from build123d import *

# Parameters (mm, degrees)
SKETCH1_W           = 95
SKETCH1_H           = 75
BOSS_EXTRUDE1_DEPTH = 32.5
SKETCH2_W           = 90
SKETCH2_H           = 70
CUT_EXTRUDE1_DEPTH  = 30
SKETCH3_R           = 1.75
BOSS_EXTRUDE2_DEPTH = 7
SKETCH4_R           = 1
BOSS_EXTRUDE3_DEPTH = 23
SKETCH5_W           = 52.348164398
SKETCH5_H           = 12
CUT_EXTRUDE2_DEPTH  = 7
FILLET1_R           = 2.5
FILLET2_R           = 2.5
FILLET3_R           = 2.5
FILLET4_R           = 2.5
FILLET5_R           = 2.5


with BuildPart() as part:
    # Sketch1 → Boss-Extrude1 (new body)
    with BuildSketch(Plane(origin=(0, 0, 0), x_dir=(1, 0, 0), z_dir=(0, 1, 0))):
        Rectangle(SKETCH1_W, SKETCH1_H)
    extrude(amount=BOSS_EXTRUDE1_DEPTH)

    # Sketch2 → Cut-Extrude1 (cut)
    with BuildSketch(Plane(origin=(0, 32.5, 0), x_dir=(1, 0, 0), z_dir=(0, 1, 0))):
        Rectangle(SKETCH2_W, SKETCH2_H)
    extrude(amount=-CUT_EXTRUDE1_DEPTH, mode=Mode.SUBTRACT)

    # Sketch3 → Boss-Extrude2 (add)
    with BuildSketch(Plane(origin=(0, 2.5, 0), x_dir=(1, 0, 0), z_dir=(0, 1, 0))):
        with Locations(Location((-41.5, 32.5, 0), (0, 0, 270))):
            Circle(SKETCH3_R)
        with Locations(Location((41.5, 32.5, 0), (0, 0, 270))):
            Circle(SKETCH3_R)
        with Locations(Location((41.5, -32.5, 0), (0, 0, 270))):
            Circle(SKETCH3_R)
        with Locations(Location((-41.5, -32.5, 0), (0, 0, 270))):
            Circle(SKETCH3_R)
    extrude(amount=BOSS_EXTRUDE2_DEPTH)

    # Sketch4 → Boss-Extrude3 (add)
    with BuildSketch(Plane(origin=(0, 9.5, 0), x_dir=(1, 0, 0), z_dir=(0, 1, 0))):
        with Locations(Location((-41.5, 32.5, 0), (0, 0, 270))):
            Circle(SKETCH4_R)
        with Locations(Location((41.5, 32.5, 0), (0, 0, 270))):
            Circle(SKETCH4_R)
        with Locations(Location((41.5, -32.5, 0), (0, 0, 270))):
            Circle(SKETCH4_R)
        with Locations(Location((-41.5, -32.5, 0), (0, 0, 270))):
            Circle(SKETCH4_R)
    extrude(amount=BOSS_EXTRUDE3_DEPTH)

    # Sketch5 → Cut-Extrude2 (cut)
    with BuildSketch(Plane(origin=(47.5, 0, 0), x_dir=(0, 0, -1), z_dir=(1, 0, 0))):
        with Locations((-1.674082199, 15.5)):
            Rectangle(SKETCH5_W, SKETCH5_H)
    extrude(amount=-CUT_EXTRUDE2_DEPTH, mode=Mode.SUBTRACT)

    # Fillet1
    fillet1_edges = [part.edges().sort_by_distance(p)[0] for p in [
        (0, 0, -37.5),
        (47.5, 0, 0),
        (0, 0, 37.5),
        (-47.5, 0, 0),
    ]]
    fillet(fillet1_edges, radius=FILLET1_R)

    # Fillet2
    # the kernel refuses this fillet: 2.5 mm, written as the material it takes off along each edge
    with BuildSketch(Plane(origin=(45, 2.5, 35), x_dir=(0, 0, 1), z_dir=(1, 0, 0))) as fillet2_piece_1_section:
        Polygon((0, 0), (FILLET2_R, 0), (FILLET2_R, FILLET2_R), (0, FILLET2_R), align=None)
    fillet2_piece_1 = extrude(amount=FILLET2_R, mode=Mode.PRIVATE)
    fillet2_piece_1 = fillet2_piece_1 - Plane(origin=(45, 2.5, 35), x_dir=(0, 0.7071067811865475, -0.7071067811865475), z_dir=(1, 0, 0)) * Sphere(FILLET2_R, mode=Mode.PRIVATE)
    add(fillet2_piece_1, mode=Mode.SUBTRACT)
    with BuildSketch(Plane(origin=(47.5, 2.5, 37.5), x_dir=(0, 0, -1), z_dir=(0, 1, 0))) as fillet2_piece_2:
        with BuildLine():
            CenterArc((FILLET2_R, FILLET2_R), FILLET2_R, 180, 90)
            Line((0, FILLET2_R), (0, 0))
            Line((0, 0), (FILLET2_R, 0))
        make_face()
    extrude(amount=36.25, mode=Mode.SUBTRACT)

    # Fillet3
    # the kernel refuses this fillet: 2.5 mm, written as the material it takes off along each edge
    with BuildSketch(Plane(origin=(45, 2.5, -35), x_dir=(1, 0, 0), z_dir=(0, 0, -1))) as fillet3_piece_1_section:
        Polygon((0, 0), (FILLET3_R, 0), (FILLET3_R, FILLET3_R), (0, FILLET3_R), align=None)
    fillet3_piece_1 = extrude(amount=FILLET3_R, mode=Mode.PRIVATE)
    fillet3_piece_1 = fillet3_piece_1 - Plane(origin=(45, 2.5, -35), x_dir=(-0.7071067811865475, 0.7071067811865475, 0), z_dir=(0, 0, -1)) * Sphere(FILLET3_R, mode=Mode.PRIVATE)
    add(fillet3_piece_1, mode=Mode.SUBTRACT)
    with BuildSketch(Plane(origin=(47.5, 2.5, -37.5), x_dir=(-1, 0, 0), z_dir=(0, 1, 0))) as fillet3_piece_2:
        with BuildLine():
            CenterArc((FILLET3_R, FILLET3_R), FILLET3_R, 180, 90)
            Line((0, FILLET3_R), (0, 0))
            Line((0, 0), (FILLET3_R, 0))
        make_face()
    extrude(amount=36.25, mode=Mode.SUBTRACT)

    # Fillet4
    # the kernel refuses this fillet: 2.5 mm, written as the material it takes off along each edge
    with BuildSketch(Plane(origin=(-45, 2.5, -35), x_dir=(-1, 0, 0), z_dir=(0, 0, -1))) as fillet4_piece_1_section:
        Polygon((0, 0), (FILLET4_R, 0), (FILLET4_R, -FILLET4_R), (0, -FILLET4_R), align=None)
    fillet4_piece_1 = extrude(amount=FILLET4_R, mode=Mode.PRIVATE)
    fillet4_piece_1 = fillet4_piece_1 - Plane(origin=(-45, 2.5, -35), x_dir=(0.7071067811865475, 0.7071067811865475, 0), z_dir=(0, 0, -1)) * Sphere(FILLET4_R, mode=Mode.PRIVATE)
    add(fillet4_piece_1, mode=Mode.SUBTRACT)
    with BuildSketch(Plane(origin=(-47.5, 2.5, -37.5), x_dir=(1, 0, 0), z_dir=(0, 1, 0))) as fillet4_piece_2:
        with BuildLine():
            CenterArc((FILLET4_R, -FILLET4_R), FILLET4_R, 90, 90)
            Line((0, -FILLET4_R), (0, 0))
            Line((0, 0), (FILLET4_R, 0))
        make_face()
    extrude(amount=36.25, mode=Mode.SUBTRACT)

    # Fillet5
    # the kernel refuses this fillet: 2.5 mm, written as the material it takes off along each edge
    with BuildSketch(Plane(origin=(-45, 2.5, 35), x_dir=(0, 0, 1), z_dir=(-1, 0, 0))) as fillet5_piece_1_section:
        Polygon((0, 0), (FILLET5_R, 0), (FILLET5_R, -FILLET5_R), (0, -FILLET5_R), align=None)
    fillet5_piece_1 = extrude(amount=FILLET5_R, mode=Mode.PRIVATE)
    fillet5_piece_1 = fillet5_piece_1 - Plane(origin=(-45, 2.5, 35), x_dir=(0, 0.7071067811865475, -0.7071067811865475), z_dir=(-1, 0, 0)) * Sphere(FILLET5_R, mode=Mode.PRIVATE)
    add(fillet5_piece_1, mode=Mode.SUBTRACT)
    with BuildSketch(Plane(origin=(-47.5, 2.5, 37.5), x_dir=(0, 0, -1), z_dir=(0, 1, 0))) as fillet5_piece_2:
        with BuildLine():
            CenterArc((FILLET5_R, -FILLET5_R), FILLET5_R, 90, 90)
            Line((0, -FILLET5_R), (0, 0))
            Line((0, 0), (FILLET5_R, 0))
        make_face()
    extrude(amount=36.25, mode=Mode.SUBTRACT)


solid = part.part
The model under review builds one solid part; all positions refer to its coordinate system, in mm. A direction names the side the tool comes from. Give positions to 0.01 mm unless a question says otherwise; leave off trailing zeros. Order: outer loops, then holes, each group sorted by start corner. A loop starts at its lowest first (then second) coordinate and runs counter-clockwise, first axis right, second up. Notation, with made-up numbers: M 24,-37.75 L 82,-37.75 A8 ccw 82,-25.75 Z; hole C 11,30.5 d8. An arc over 180 degrees is marked long. Use one line per item in the form item = value. Start each with the question number.
Item 1: The part is to be moulded in two halves that separate along Z. For faces 4 (the cylindrical face through (1, 1, -37)), 5 (the cylindrical face through (46.748, 17.29, 36.787)), 6 (the flat face through (-4, 32.5, 36)), 7 (the flat face through (46, 15, 27.848)), say which applies: pulls with the +Z half, pulls with the -Z half, needs draft (parallel to the pull), parting line crosses it, or undercut.
Item 2: For faces 1 (the cylindrical face through (42.49, 20.84, 32.37)), 2 (the flat face through (42, 32.5, -33)), 3 (the flat face through (46, 21.5, 2)), list the 3-axis set-ups (+Z, -Z, +X, -X, +Y, -Y) from which the entire face can be reached by the end or side of a thin tool; tool diameter is ignored.
Item 3: We need section B-B on z = 26.5. Give the boundary of the cut face in (x, y), plus the area to 3 significant figures.
Item 4: We need section D-D on x = -32.5. Give the boundary of the cut face in (y, z), plus the area to 3 significant figures.
Item 5: We need section C-C on y = 17. Give the boundary of the cut face in (x, z), plus the area to 3 significant figures.
Item 6: Insertion check: pin 1 Ø2 at (x, y) = (47, 18) entering from -Z; pin 2 Ø1.2 at (x, y) = (46, 16) entering from +Z; pin 3 Ø2 at (x, z) = (46.5, 4.5) entering from -Y. Each pin has a flat end and moves straight along its axis. Give the tip position at first contact, or say it passes through.
Item 7: We need section A-A on y = 30.5. Give the boundary of the cut face in (x, z).
Item 8: To check wall thickness, follow line 1 along Z through (x, y) = (4, 24); line 2 along X through (y, z) = (4, 0.5); line 3 along Y through (x, z) = (41, 23). State the ranges of each line that lie inside material, in increasing order. Write a range as from..to.
Completed:
q1.face_4 = pulls with the -Z half
q1.face_5 = pulls with the +Z half
q1.face_6 = needs draft
q1.face_7 = undercut
q2.face_1 = +Y
q2.face_2 = +Z, -Z, +X, -X, +Y
q2.face_3 = +X
q3.outline = M -47.5,2.5 A2.5 ccw -45,0 L 45,0 A2.5 ccw 47.5,2.5 L 47.5,9.5 L 45,9.5 L 45,2.5 L -45,2.5 L -45,32.5 L -47.5,32.5 Z; M 45,21.5 L 47.5,21.5 L 47.5,32.5 L 45,32.5 Z
q3.area = 355 mm²
q4.outline = M 0,-35 A2.5 ccw 2.5,-37.5 L 32.5,-37.5 L 32.5,-35 L 2.5,-35 L 2.5,35 L 32.5,35 L 32.5,37.5 L 2.5,37.5 A2.5 ccw 0,35 Z
q4.area = 335 mm²
q5.outline = M -47.5,-35 A2.5 ccw -45,-37.5 L 45,-37.5 A2.5 ccw 47.5,-35 L 47.5,-24.5 L 45,-24.5 L 45,-35 L -45,-35 L -45,35 L 45,35 L 45,27.85 L 47.5,27.85 L 47.5,35 A2.5 ccw 45,37.5 L -45,37.5 A2.5 ccw -47.5,35 Z; C -41.5,-32.5 d2; C -41.5,32.5 d2; C 41.5,-32.5 d2; C 41.5,32.5 d2
q5.area = 701 mm²
q6.pin_1 = -37.29
q6.pin_2 = 37.47
q6.pin_3 = 0.05
q7.outline = M -47.5,-35 A2.5 ccw -45,-37.5 L 45,-37.5 A2.5 ccw 47.5,-35 L 47.5,35 A2.5 ccw 45,37.5 L -45,37.5 A2.5 ccw -47.5,35 Z; C -41.5,-32.5 d2; C -41.5,32.5 d2; C 41.5,-32.5 d2; C 41.5,32.5 d2; hole M -45,-35 L 45,-35 L 45,35 L -45,35 Z
q8.line_1 = -37.5..-35, 35..37.5
q8.line_2 = -47.5..-45, 45..47.5
q8.line_3 = 0..2.5
